Build history of the part. All positions in model axes, mm. Coordinates: 2 decimals unless noted, no trailing zeros. Write each loop counter-clockwise with the first axis right and the second up, starting at its lowest first coordinate (ties: lowest second). Pieces come first, ordered by that corner, then holes.
```python
from build123d import *

# Parameters (mm, degrees)
PAD_DEPTH    = 2
PAD001_DEPTH = 116
PAD002_DEPTH = 2


with BuildPart() as part:
    # Sketch → Pad (new body)
    with BuildSketch(Plane.YZ):
        with BuildLine():
            Line((-9.7, 0), (0, 0))
            Line((0, 0), (0, -10.3))
            ThreePointArc((-1.707, -10.992), (-0.624263, -11.211473), (0, -10.3))
            Line((-9.406686, -3.292314), (-1.707, -10.992))
            ThreePointArc((-9.7, -2.59), (-9.62277, -2.970153), (-9.406686, -3.292314))
            Line((-9.7, 0), (-9.7, -2.59))
        make_face()
    extrude(amount=PAD_DEPTH)

    # Sketch001 (on Face8 of Pad) → Pad001 (join)
    with BuildSketch(Plane.YZ.offset(2)):
        with BuildLine():
            Line((0, -3), (0, -10.3))
            ThreePointArc((-1.707, -10.992), (-0.624263, -11.211473), (0, -10.3))
            Line((-8.9902, -3.7088), (-1.707, -10.992))
            ThreePointArc((-8.3, -2), (-9.211954, -2.625443), (-8.9902, -3.7088))
            Line((-8.3, -2), (-1, -2))
            ThreePointArc((0, -3), (-0.292893, -2.292893), (-1, -2))
        make_face()
    extrude(amount=PAD001_DEPTH)

    # Sketch002 (on Face9 of Pad001) → Pad002 (join)
    with BuildSketch(Plane.YZ.offset(118)):
        with BuildLine():
            Line((0, 0), (0, -10.3))
            ThreePointArc((-1.707, -10.992), (-0.624263, -11.211473), (0, -10.3))
            Line((-9.406686, -3.292314), (-1.707, -10.992))
            ThreePointArc((-9.7, -2.59), (-9.62277, -2.970153), (-9.406686, -3.292314))
            Line((-9.7, 0), (-9.7, -2.59))
            Line((0, 0), (-9.7, 0))
        make_face()
    extrude(amount=PAD002_DEPTH)


solid = part.part
```
1. Saw through at A-A on x = 87. List the corners of the cut face in (y, z), plus the area to 3 significant figures.
Computed values:
outline: (-8.99, -3.71) - (-1.71, -10.99) arc R1 ccw to (0, -10.3) - (0, -3) arc R1 ccw to (-1, -2) - (-8.3, -2) arc R1 ccw to start
area: 54.5 mm2
2. Saw through at B-B on y = -6. List the corners of the cut face in (x, z), plus the area to 3 significant figures.
Computed values:
outline: (0, -6.7) - (120, -6.7) - (120, 0) - (118, 0) - (118, -2) - (2, -2) - (2, 0) - (0, 0) - close
area: 572 mm2
3. Saw through at C-C on z = -5. List the corners of the cut face in (x, y).
Computed values:
outline: (0, -7.7) - (120, -7.7) - (120, 0) - (0, 0) - close
4. Probe line 1 along X through (y, z) = (-5.75, -1); line 2 along Z through (x, y) = (38.5, -3); line 3 along Y through (x, z) = (58.5, -3). List the from-to ranges inside material, lowest first.
Computed values:
line 1: x = 0 to 2, 118 to 120
line 2: z = -9.7 to -2
line 3: y = -9.28 to 0
5. Flat gauge pins, fed straight in: pin 1 (1.1 mm diameter, centred on y = -4, z = -1.5, fed in from -X); pin 2 (3 mm diameter, centred on x = 21.5, y = -3.5, fed in from +Z); pin 3 (5 mm diameter, centred on x = 97.5, y = -7, fed in from -Z). Where does each tip first touch, or does it go through?
Computed values:
pin 1: stops at x = 0
pin 2: stops at z = -2
pin 3: stops at z = -8.2
6. Mould opens along X. For faces 1 (the face through (59, -5, -2)), 2 (the face through (120, -4, -4)), 3 (the face through (1, -5, 0)) say: +X half, -X half, draft (parallel to the pull), parting line (faces both ways), or undercut.
Computed values:
face 1: undercut
face 2: +X half
face 3: draft
